The drawing under review shows one solid part. Ordinate dimensions are in mm from its lowest x, y, z. A direction names the side the tool comes from. Give positions to 0.01 mm unless a question says otherwise; leave off trailing zeros. Order: outer loops, then holes, each group sorted by start corner. A loop starts at its lowest first (then second) coordinate and runs counter-clockwise, first axis right, second up. Notation, with made-up numbers: (65, 77.25) -> (121, 77.25) arc R21 cw to (121, 114.25) -> close; hole circle Ø11 at (18.25, 48). An arc over 180 degrees is marked (long way). Return JSON: item names as keys, results as strings. Group by question number.
1) To check wall thickness, follow line 1 along Z through (x, y) = (7.25, 3.25); line 2 along X through (y, z) = (4, 1.25); line 3 along X through (y, z) = (2.5, 6.5). State the ranges of each line that lie inside material, in increasing order.
2) Add section C-C (x = 3.75). Give the boundary of the cut face in (y, z) (3 decimals), then the cut area to 3 significant figures.
3) Add section B-B (y = 3.75). Give the boundary of the cut face in (x, z) (3 decimals), then the cut area to 3 significant figures.
4) For the marked faces 1 and 2, list the 3-axis set-ups (+Z, -Z, +X, -X, +Y, -Y) from which the entire face can be reached by the end or side of a thin tool; tool diameter is ignored.
5) Add section D-D (y = 2.5). Give the boundary of the cut face in (x, z), then the cut area to 3 significant figures.
6) Insertion check: P1, Ø3, axis at y = 1.5, z = 0.5, coming from the +X side; P2, Ø2, axis at x = 5.5, z = 4.5, coming from the +Y side; P3, Ø1.6, axis at y = 4.5, z = 5.5, coming from the +X side (3 decimals). Each pin has a flat end and moves straight along its axis. Give the tip position at first contact, or say it passes through.
7) Add section A-A (z = 6.75). Give the boundary of the cut face in (x, y) (3 decimals).
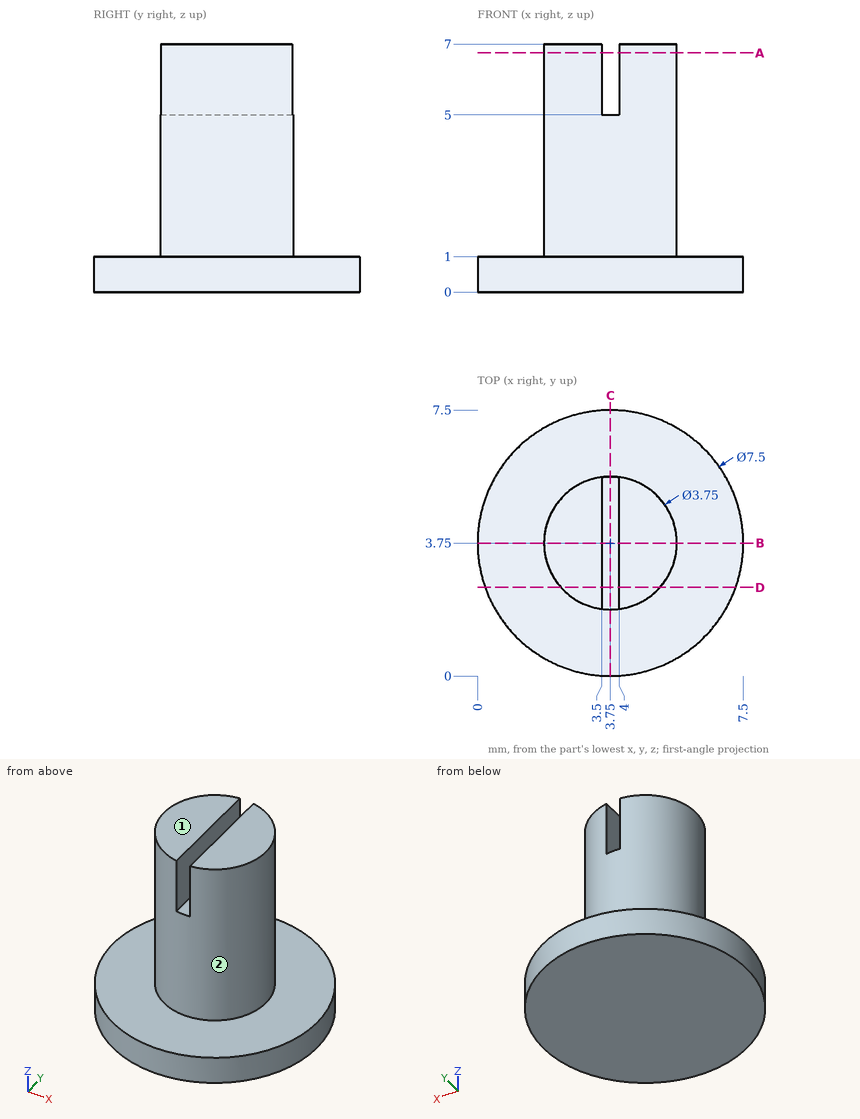
Evaluation:
{
 "1": {"line 1": "0 to 1", "line 2": "1.89 to 5.61", "line 3": "2.35 to 3.5, 4 to 5.15"},
 "2": {"outline": "(0, 0) -> (7.5, 0) -> (7.5, 1) -> (5.625, 1) -> (5.625, 5) -> (1.875, 5) -> (1.875, 1) -> (0, 1) -> close", "area": "22.5 mm^2"},
 "3": {"outline": "(0, 0) -> (7.5, 0) -> (7.5, 1) -> (5.625, 1) -> (5.625, 7) -> (4, 7) -> (4, 5) -> (3.5, 5) -> (3.5, 7) -> (1.875, 7) -> (1.875, 1) -> (0, 1) -> close", "area": "29.0 mm^2"},
 "4": {"face 1": "+Z, +X, -X, +Y, -Y", "face 2": "+Z"},
 "5": {"outline": "(0.21, 0) -> (7.29, 0) -> (7.29, 1) -> (5.15, 1) -> (5.15, 7) -> (4, 7) -> (4, 5) -> (3.5, 5) -> (3.5, 7) -> (2.35, 7) -> (2.35, 1) -> (0.21, 1) -> close", "area": "22.8 mm^2"},
 "6": {"P1": "x = 7.42", "P2": "y = 5.47", "P3": "x = 5.625"},
 "7": {"outline": "(3.5, 1.892) -> (3.5, 5.608) arc R1.875 ccw to start; (4, 1.892) arc R1.875 ccw to (4, 5.608) -> close"}
}
